```python
from build123d import *

# Parameters (mm, degrees)
F0_W     = 45
F0_H     = 20
F1_DEPTH = 1.6
F2_R     = 8
F3_DEPTH = 12


with BuildPart() as f1:
    # F0 (on Front) → F1 (new body)
    with BuildSketch(Plane.XZ):
        Rectangle(F0_W, F0_H)
    extrude(amount=F1_DEPTH)

    # F2 (on Front) → F3 (join)
    with BuildSketch(Plane.XZ):
        with Locations((-13.5, 0)):
            Circle(F2_R)
        with BuildLine():
            ThreePointArc((21.5, 0), (13.5, 8), (5.5, 0))
            ThreePointArc((5.5, 0), (13.5, -8), (21.5, 0))
        make_face()
    extrude(amount=F3_DEPTH)


solid = f1.part
```
For this review, take the finished solid that the model builds, in its own axes (mm). A direction names the side the tool comes from. Coordinates: 2 decimals unless noted, no trailing zeros. Loops run counter-clockwise (first coordinate to the right, second up) from the corner with the lowest first, then second, coordinate; pieces in that order, holes last.
1. For line 1 (Y direction, x = 2, z = -3); line 2 (X direction, y = -7, z = 5.5); line 3 (X direction, y = -7.5, z = -2), list the stretches that pass through material, from the lowest coordinate up.
2. Add section C-C, the plane z = 2.25. Give the boundary of the cut face in (x, y), then the cut area to 3 significant figures.
3. Add section A-A, the plane x = 13.5. Give the boundary of the cut face in (y, z).
4. Mouldability with a two-part tool opening along X and no side actions: class faces 1 (the flat face through (0, -1, -10)), 2 (the flat face through (-22.5, -1, 0)), 3 (the cylindrical face through (15.23, -6.73, 7.81)) as +X half, -X half, draft (parallel to the pull), parting line (faces both ways), or undercut.
5. Add section B-B, the plane z = 0. Give the boundary of the cut face in (x, y), then the cut area to 3 significant figures.
6. For faces 4 (the flat face through (0, -1, 10)), 5 (the cylindrical face through (-15.23, -6.73, -7.81)), list the 3-axis set-ups (+Z, -Z, +X, -X, +Y, -Y) from which the entire face can be reached by the end or side of a thin tool; tool diameter is ignored.
7. Insertion check: P1, Ø3, axis at x = 10.5, y = -6, coming from the +Z side; P2, Ø3, axis at y = -8.5, z = -1.5, coming from the -X side; P3, Ø4, axis at y = -6, z = 5, coming from the +X side; P4, Ø4, axis at x = -17, z = 2.5, coming from the +Y side. Each pin has a flat end and moves straight along its axis. Give the tip position at first contact, or say it passes through.
8. Add section D-D, the plane x = 20. Give the boundary of the cut face in (y, z).
Result:
1. line 1: y = -1.6 to 0
1. line 2: x = -19.31 to -7.69, 7.69 to 19.31
1. line 3: x = -21.25 to -5.75, 5.75 to 21.25
2. outline: (-22.5, -1.6) - (-21.18, -1.6) - (-21.18, -12) - (-5.82, -12) - (-5.82, -1.6) - (5.82, -1.6) - (5.82, -12) - (21.18, -12) - (21.18, -1.6) - (22.5, -1.6) - (22.5, 0) - (-22.5, 0) - close
2. area: 391 mm2
3. outline: (-12, -8) - (-1.6, -8) - (-1.6, -10) - (0, -10) - (0, 10) - (-1.6, 10) - (-1.6, 8) - (-12, 8) - close
4. face 1: draft
4. face 2: -X half
4. face 3: undercut
5. outline: (-22.5, -1.6) - (-21.5, -1.6) - (-21.5, -12) - (-5.5, -12) - (-5.5, -1.6) - (5.5, -1.6) - (5.5, -12) - (21.5, -12) - (21.5, -1.6) - (22.5, -1.6) - (22.5, 0) - (-22.5, 0) - close
5. area: 405 mm2
6. face 4: +Z, +X, -X, +Y, -Y
6. face 5: -Y
7. P1: stops at z = 7.86
7. P2: stops at x = -21.5
7. P3: stops at x = 20.92
7. P4: stops at y = 0
8. outline: (-12, -4.66) - (-1.6, -4.66) - (-1.6, -10) - (0, -10) - (0, 10) - (-1.6, 10) - (-1.6, 4.66) - (-12, 4.66) - close
